Part model, mm, in its own coordinate system. A direction names the side the tool comes from. Coordinates: 2 decimals unless noted, no trailing zeros. Loops run counter-clockwise (first coordinate to the right, second up) from the corner with the lowest first, then second, coordinate; pieces in that order, holes last. Notation, with made-up numbers: (20.5, -17) -> (78.5, -17) arc R26 ccw to (78.5, 22) -> close; hole circle Ø7 at (-5, 80.25). An arc over 180 degrees is marked (long way). One line per question, with ' | ' between items. Start each with the question number.
1) Drop flat-ended pins along their axis: pin 1 (3 mm diameter, centred on y = -57, z = -2, fed in from -X); pin 2 (3 mm diameter, centred on y = -62, z = 2, fed in from +X); pin 3 (3 mm diameter, centred on x = -59, z = -1, fed in from +Y); pin 4 (1 mm diameter, centred on y = 41.5, z = 7, fed in from +X). Give the stop position or say it passes through.
2) Cut at A-A (y = 0). List the corners of the cut face in (x, z).
3) Probe L1, parallel to X at y = 60, z = 0.25; L2, parallel to Z at x = 40, y = 18.5; L3, parallel to Y at x = 0, z = 3.25. List the from-to ranges inside material, lowest first. Write a range as from..to.
4) Cut at D-D (x = -49). List the corners of the cut face in (y, z), plus the area to 3 significant figures.
5) Cut at C-C (x = 0). List the corners of the cut face in (y, z) (3 decimals).
6) 3-axis set-ups, long thin cutter, end or side, ignore diameter. For faces 5 (the face through (-2.38, -10.74, 9.93)), 6 (the face through (19.792, -56, 0)), 7 (the face through (-9.792, 64, 0)), 8 (the face through (-19.792, -56, 0)), 9 (the face through (-56, 19.792, 0)): which of +Z, -Z, +X, -X, +Y, -Y reach the whole face in a straight line?
7) Two-plate mould, pull along Y, no slides. Class faces 1 (the face through (43.317, 0.215, 0.07)), 2 (the face through (-64, -9.792, 0)), 3 (the face through (-25.5, -25.8, -0.1)), 4 (the face through (5, -5, 15)): released by +Y, released by -Y, zero draft, split by the parting line, or undercut.
from build123d import *

# Parameters (mm, degrees)
ESQUISSE1_R                  = 75
BOSS_EXTRU_1_DEPTH           = 5
ENL_V_MAT_EXTRU_1_DEPTH      = 20
R_P_TITION_CIRCULAIRE1_COUNT = 4
ESQUISSE3_W                  = 52.549672888
ESQUISSE3_H                  = 52.549672888
ENL_V_MAT_EXTRU_2_DEPTH      = 20
R_P_TITION_CIRCULAIRE2_COUNT = 4
CONG_1_R                     = 20
ENL_V_MAT_EXTRU_3_DEPTH      = 106.632580986
ENL_V_MAT_EXTRU_3_DEPTH_BACK = 106.632580986
ESQUISSE6_R                  = 11
BOSS_EXTRU_2_DEPTH           = 10
ESQUISSE7_R                  = 2.175
ENL_V_MAT_EXTRU_4_DEPTH      = 14


with BuildPart() as part:
    # Esquisse1 → Boss.-Extru.1 (new, symmetric)
    with BuildSketch(Plane.XY):
        Circle(ESQUISSE1_R)
    extrude(amount=BOSS_EXTRU_1_DEPTH, both=True)

    # Esquisse2 → Enlèv. mat.-Extru.1 (cut)
    with BuildSketch(Plane.XY.offset(5)):
        with BuildLine():
            Line((-53.106036975, 9.791778038), (-74.358059972, 9.791778038))
            ThreePointArc((-74.358059972, 9.791778038), (-75, 0), (-74.358059972, -9.791778038))
            Line((-74.358059972, -9.791778038), (-53.106036975, -9.791778038))
            ThreePointArc((-53.106036975, -9.791778038), (-43.314258937, 0), (-53.106036975, 9.791778038))
        make_face()
    enl_v_mat_extru_1 = extrude(amount=-ENL_V_MAT_EXTRU_1_DEPTH, mode=Mode.SUBTRACT)

    # Répétition circulaire1: Enlèv. mat.-Extru.1 ×4 about axis
    r_p_tition_circulaire1_axis = Axis((0, 0, 0), (0, 0, 1))
    for i in range(1, R_P_TITION_CIRCULAIRE1_COUNT):
        add(enl_v_mat_extru_1.rotate(r_p_tition_circulaire1_axis, i * 360 / R_P_TITION_CIRCULAIRE1_COUNT), mode=Mode.SUBTRACT)

    # Esquisse3 → Enlèv. mat.-Extru.2 (cut)
    with BuildSketch(Plane.XY.offset(5)):
        with Locations((-46.066614482, 46.066614482)):
            Rectangle(ESQUISSE3_W, ESQUISSE3_H)
    enl_v_mat_extru_2 = extrude(amount=-ENL_V_MAT_EXTRU_2_DEPTH, mode=Mode.SUBTRACT)

    # Répétition circulaire2: Enlèv. mat.-Extru.2 ×4 about axis
    r_p_tition_circulaire2_axis = Axis((0, 0, 0), (0, 0, 1))
    for i in range(1, R_P_TITION_CIRCULAIRE2_COUNT):
        add(enl_v_mat_extru_2.rotate(r_p_tition_circulaire2_axis, i * 360 / R_P_TITION_CIRCULAIRE2_COUNT), mode=Mode.SUBTRACT)

    # Congé1
    cong_1_edges = [part.edges().sort_by_distance(p)[0] for p in [
        (-19.791778038, -19.791778038, 0),
        (19.791778038, -19.791778038, 0),
        (19.791778038, 19.791778038, 0),
        (-19.791778038, 19.791778038, 0),
    ]]
    fillet(cong_1_edges, radius=CONG_1_R)

    # Esquisse4 → Enlèv. mat.-Extru.3 (cut, two sides: drawn at the far end of the back side and taken through both)
    with BuildSketch(Plane.XY.offset(5).offset(-ENL_V_MAT_EXTRU_3_DEPTH_BACK)):
        with BuildLine():
            Line((-3.31662479, 5), (3.31662479, 5))
            ThreePointArc((3.31662479, 5), (0, -6), (-3.31662479, 5))
        make_face()
    extrude(amount=ENL_V_MAT_EXTRU_3_DEPTH + ENL_V_MAT_EXTRU_3_DEPTH_BACK, mode=Mode.SUBTRACT)

    # Esquisse6 → Boss.-Extru.2 (add)
    with BuildSketch(Plane.XY.offset(5)):
        Circle(ESQUISSE6_R)
        with BuildLine():
            Line((-3.31662479, 5), (3.31662479, 5))
            ThreePointArc((3.31662479, 5), (0, -6), (-3.31662479, 5))
        make_face(mode=Mode.SUBTRACT)
    extrude(amount=BOSS_EXTRU_2_DEPTH)

    # Esquisse7 → Enlèv. mat.-Extru.4 (cut)
    with BuildSketch(Plane(origin=(0, 0, 0), x_dir=(1, 0, 0), z_dir=(0, 1, 0))):
        with Locations(Location((0, -10, 0), (0, 0, 90))):
            Circle(ESQUISSE7_R)
    extrude(amount=ENL_V_MAT_EXTRU_4_DEPTH, mode=Mode.SUBTRACT)


solid = part.part
Reported:
1) pin 1: stops at x = -19.79 | pin 2: stops at x = 19.79 | pin 3: stops at y = 19.79 | pin 4: passes through
2) outline: (-43.31, -5) -> (-6, -5) -> (-6, 15) -> (-11, 15) -> (-11, 5) -> (-43.31, 5) -> close; (6, -5) -> (43.31, -5) -> (43.31, 5) -> (11, 5) -> (11, 15) -> (6, 15) -> close
3) L1: x = -19.79..-9.79, 9.79..19.79 | L2: z = -5..5 | L3: y = -43.31..-6, 5..43.31
4) outline: (-19.79, -5) -> (-8.89, -5) -> (-8.89, 5) -> (-19.79, 5) -> close; (8.89, -5) -> (19.79, -5) -> (19.79, 5) -> (8.89, 5) -> close | area: 218 mm²
5) outline: (-43.314, -5) -> (-6, -5) -> (-6, 15) -> (-11, 15) -> (-11, 5) -> (-43.314, 5) -> close; (5, -5) -> (43.314, -5) -> (43.314, 5) -> (11, 5) -> (11, 7.825) -> (5, 7.825) -> close; (5, 12.175) -> (11, 12.175) -> (11, 15) -> (5, 15) -> close
6) face 5: +Z | face 6: +Z, -Z, +X, -Y | face 7: +Z, -Z, +Y | face 8: +Z, -Z, -X, -Y | face 9: +Z, -Z, -X, +Y
7) face 1: undercut | face 2: undercut | face 3: released by -Y | face 4: zero draft
